Solid Edge part; units mm, degrees
sketch "Sketch1" plane through (10.8674, 0, 10.8674) normal (0, -1, 0) x (1, 0, 0)
  circle A0 centre (-10.8674, -10.8674) radius 15
extrude "Protrusion1" add sketch "Sketch1" against normal blind 500
chamfer "Chamfer" distance 1 angle 45 1 edges at (-15, 0, 0)
sketch "Sketch2" plane through (0, 250.5, 15) normal (0, 0, 1) x (0, -1, 0)
  line L0 (203.5, -4) -> (240.5, -4)
  arc A0 (240.5, 4) -> (240.5, -4) centre (240.5, 0) cw
  line L1 (240.5, 4) -> (203.5, 4)
  arc A1 (203.5, 4) -> (203.5, -4) centre (203.5, 0) ccw
extrude "KeySlot_Wheel_Hub" cut sketch "Sketch2" against normal blind 4
mirror "Mirror1" about plane through (0, 500, 0) normal (0, 1, 0) of "Protrusion1", "KeySlot_Wheel_Hub"
sketch "Sketch3" plane through (-2.7141, 250.8352, 11) normal (0, 0, 1) x (0, -1, 0)
  line L0 (-517.1648, -4) -> (-500.1648, -4)
  arc A0 (-500.1648, 4) -> (-500.1648, -4) centre (-500.1648, 0) cw
  line L1 (-500.1648, 4) -> (-517.1648, 4)
  arc A1 (-517.1648, 4) -> (-517.1648, -4) centre (-517.1648, 0) ccw
extrude "Cutout2" cut sketch "Sketch3" along normal blind 61.758
sketch "Sketch4" plane through (-1.1004, 261.9084, 11) normal (0, 0, 1) x (0, -1, 0)
  line L0 (-99.0916, -4) -> (-82.0916, -4)
  arc A0 (-82.0916, 4) -> (-82.0916, -4) centre (-82.0916, 0) cw
  line L1 (-82.0916, 4) -> (-99.0916, 4)
  arc A1 (-99.0916, 4) -> (-99.0916, -4) centre (-99.0916, 0) ccw
extrude "KeySlot_Chain_Sprocket_Hub" cut sketch "Sketch4" along normal blind 21.355
properties material "Steel"
For this review, take the finished solid that the model builds, in its own axes (mm). Give positions to 0.01 mm unless a question says otherwise; leave off trailing zeros. Order: outer loops, then holes, each group sorted by start corner. A loop starts at its lowest first (then second) coordinate and runs counter-clockwise, first axis right, second up. Notation, with made-up numbers: M 22,-19 L 54,-19 A15 cw 54,0 Z; hole C -16,73 d10. An arc over 180 degrees is marked long. Answer in a Markdown table with one row per item. Add a question column.
(1) For pin 1 (4.5 mm diameter, centred on y = 763.5, z = 13.5, fed in from -X); pin 2 (2 mm diameter, centred on y = 416.5, z = -11.5, fed in from -X); pin 3 (3 mm diameter, centred on y = 476, z = -9.5, fed in from +X), all flat-tipped, find the tip position at first contact; note any pin that passes through.
(2) Consider section B-B on y = 759.5. State the section outline as (x, z) points, and give its area (3 significant figures).
(3) Consider section A-A on y = 923.5. State the section outline as (x, z) points, and give its area (3 significant figures).
(4) Wall thickness on probe 1 along Z at (x, y) = (-2, 855.5); probe 2 along Z at (x, y) = (0.5, 716): over which ranges is each line inside the solid? List them lowest first. Write a range as [from, to].
Evaluation:
| question | item | result |
|---|---|---|
| 1 | pin 1 | stops at x = -9.92 |
| 1 | pin 2 | stops at x = -10.71 |
| 1 | pin 3 | stops at x = 12.69 |
| 2 | outline | M -6.71,11 L -6.71,13.41 A15 ccw long 1.29,14.94 L 1.29,11 Z |
| 2 | area | 678 mm^2 |
| 3 | outline | C 0,0 d30 |
| 3 | area | 707 mm^2 |
| 4 | probe 1 | z = [-14.87, 14.87] |
| 4 | probe 2 | z = [-14.99, 14.99] |
